from build123d import *

# Parameters (mm, degrees)
F0_W          = 100
F0_H          = 30
F1_DEPTH      = 30
F3_R          = 10.5
F4_DEPTH      = 100
F5_W          = 30
F5_H          = 30
F6_DEPTH      = 35
F2_W          = 30
F2_H          = 30
F7_DEPTH      = 35
F9_DEPTH      = 5
F10_DEPTH     = 35
F11_DEPTH     = 30
F12_DEPTH     = 5
F13_R         = 10.5
F14_DEPTH     = 50
F15_R         = 10.5
F16_DEPTH     = 50
F17_T4_DEPTH  = 78.1749423251
F17_T9_DEPTH  = 78.1749423251
F17_T14_DEPTH = 60.7168298797
F17_T19_DEPTH = 60.7168298797
F18_T4_DEPTH  = 52.8584149398
F18_T9_DEPTH  = 60.7168298797
F18_T15_DEPTH = 60.7168298797
F18_T21_DEPTH = 60.7168298797
F18_T27_DEPTH = 60.7168298797
F18_T33_DEPTH = 52.8584149398


# Not quite as in the source:
# - a fillet or chamfer that OpenCascade refuses, or shapes differently, is made with other operations: its cross-section is extruded or revolved along the edge and cut away or added


with BuildPart() as f1:
    # F0 (on Top) → F1 (new body)
    with BuildSketch(Plane.XY):
        Rectangle(F0_W, F0_H)
    extrude(amount=F1_DEPTH)

    # F3 (on face) → F4 (cut)
    with BuildSketch(Plane(origin=(-50, 0, 0), x_dir=(0, -1, 0), z_dir=(-1, 0, 0))):
        with Locations((0, 15)):
            Circle(F3_R)
    extrude(amount=-F4_DEPTH, mode=Mode.SUBTRACT)

    # F5 (on face) → F6 (join)
    with BuildSketch(Plane.XZ.offset(15)):
        with Locations((0, 15)):
            Rectangle(F5_W, F5_H)
    extrude(amount=F6_DEPTH)

    # F2 (on face) → F7 (join)
    with BuildSketch(Plane.XY.offset(30)):
        Rectangle(F2_W, F2_H)
    extrude(amount=F7_DEPTH)

    # F8 (on face) → F9 (join)
    with BuildSketch(Plane(origin=(-15, 0, 0), x_dir=(0, -1, 0), z_dir=(-1, 0, 0))):
        Polygon((15, 65), (15, 30), (24.8667589854, 63.5804566247), (-2.7490875563, 71.6946673709), (-4.7161444721, 65), align=None)
        Polygon((-15, 30), (15, 30), (15, 65), (-4.7161444721, 65), align=None)
    extrude(amount=F9_DEPTH)

    # F10 (cut, through all): a face of the model
    f10_faces = [f1.faces().sort_by_distance(p)[0] for p in [
        (0, 0, 65),
    ]]
    extrude(f10_faces, amount=-F10_DEPTH, mode=Mode.SUBTRACT)

    # F8 (on face) → F11 (join)
    with BuildSketch(Plane(origin=(-15, 0, 0), x_dir=(0, -1, 0), z_dir=(-1, 0, 0))):
        Polygon((-15, 30), (15, 30), (15, 65), (-4.7161444721, 65), align=None)
        Polygon((15, 65), (15, 30), (24.8667589854, 63.5804566247), (-2.7490875563, 71.6946673709), (-4.7161444721, 65), align=None)
    extrude(amount=-F11_DEPTH)

    # F12 (cut): a face of the model
    f12_faces = [f1.faces().sort_by_distance(p)[0] for p in [
        (-20, -5.0118640534, 48.8916696379),
    ]]
    extrude(f12_faces, amount=-F12_DEPTH, mode=Mode.SUBTRACT)

    # F13 (on face) → F14 (cut)
    with BuildSketch(Plane.XZ.offset(50)):
        with Locations((0, 15)):
            Circle(F13_R)
    extrude(amount=-F14_DEPTH, mode=Mode.SUBTRACT)

    # F15 (on face) → F16 (cut)
    with BuildSketch(Plane(origin=(0, -19.1730464608, 65.2534085396), x_dir=(1, 0, 0), z_dir=(0, -0.2819073996, 0.9594416178))):
        with Locations((0, 8.4572219875)):
            Circle(F15_R)
    extrude(amount=-F16_DEPTH, mode=Mode.SUBTRACT)

    # F17: chamfer of 5 on 4 edges, made by hand


with BuildPart() as f17_tool2:
    # F17_s3 → F17_t4 (new body)
    with BuildSketch(Plane(origin=(0, -22.7979287792, 77.5903069724), x_dir=(1, 0, 0), z_dir=(0, 0.2819073996, -0.9594416178))):
        Polygon((-10, -22.8488462553), (-15, -17.8488462553), (-15, -22.8488462553), align=None)
    extrude(amount=F17_T4_DEPTH)

    split(bisect_by=Plane.XY.offset(30), keep=Keep.TOP)


with BuildPart() as f1_1:
    add(f1.part)

    # F17_t1: cut F17_tool2
    add(f17_tool2.part, mode=Mode.SUBTRACT)


with BuildPart() as f17_tool7:
    # F17_s8 → F17_t9 (new body)
    with BuildSketch(Plane(origin=(0, -22.7979287792, 77.5903069724), x_dir=(1, 0, 0), z_dir=(0, 0.2819073996, -0.9594416178))):
        Polygon((15, -17.8488462553), (10, -22.8488462553), (15, -22.8488462553), align=None)
    extrude(amount=F17_T9_DEPTH)

    split(bisect_by=Plane.XY.offset(30), keep=Keep.TOP)


with BuildPart() as f1_2:
    add(f1_1.part)

    # F17_t6: cut F17_tool7
    add(f17_tool7.part, mode=Mode.SUBTRACT)


with BuildPart() as f17_tool12:
    # F17_s13 → F17_t14 (new body)
    with BuildSketch(Plane(origin=(0, -5.6814051569, 19.3360534821), x_dir=(1, 0, 0), z_dir=(0, -0.2819073996, 0.9594416178))):
        Polygon((15, -0.9344022802), (10, -5.9344022802), (15, -5.9344022802), align=None)
    extrude(amount=F17_T14_DEPTH)

    split(bisect_by=Plane.XY.offset(30), keep=Keep.TOP)


with BuildPart() as f1_3:
    add(f1_2.part)

    # F17_t11: cut F17_tool12
    add(f17_tool12.part, mode=Mode.SUBTRACT)


with BuildPart() as f17_tool17:
    # F17_s18 → F17_t19 (new body)
    with BuildSketch(Plane(origin=(0, -5.6814051569, 19.3360534821), x_dir=(1, 0, 0), z_dir=(0, -0.2819073996, 0.9594416178))):
        Polygon((-10, -5.9344022802), (-15, -0.9344022802), (-15, -5.9344022802), align=None)
    extrude(amount=F17_T19_DEPTH)

    split(bisect_by=Plane.XY.offset(30), keep=Keep.TOP)


with BuildPart() as f1_4:
    add(f1_3.part)

    # F17_t16: cut F17_tool17
    add(f17_tool17.part, mode=Mode.SUBTRACT)

    # F18: chamfer of 5 on 6 edges, made by hand


with BuildPart() as f18_tool2:
    # F18_s3 → F18_t4 (new body)
    with BuildSketch(Plane.YZ.offset(62.8584149398)):
        Polygon((10, 30), (15, 25), (15, 30), align=None)
    extrude(amount=-F18_T4_DEPTH)

    split(bisect_by=Plane(origin=(16.4244231276, 15.7582750978, 4.6301664136), x_dir=(-0.6923221184, 0.7215885839, 0), z_dir=(0.7071067812, 0.6784276741, 0.1993386339)), keep=Keep.TOP)


with BuildPart() as f1_5:
    add(f1_4.part)

    # F18_t1: cut F18_tool2
    add(f18_tool2.part, mode=Mode.SUBTRACT)


with BuildPart() as f18_tool7:
    # F18_s8 → F18_t9 (new body)
    with BuildSketch(Plane.YZ.offset(-2.1415850602)):
        Polygon((-10, 30), (-15, 25), (-15, 30), align=None)
    extrude(amount=-F18_T9_DEPTH)

    split(bisect_by=Plane(origin=(-7.9672011401, -7.6440643516, -2.2460129554), x_dir=(0.6923221184, -0.7215885839, 0), z_dir=(-0.7071067812, -0.6784276741, -0.1993386339)), keep=Keep.TOP)

    split(bisect_by=Plane(origin=(-20, 0, 20), x_dir=(0, 1, 0), z_dir=(-0.7071067812, 0, 0.7071067812)), keep=Keep.TOP)


with BuildPart() as f1_6:
    add(f1_5.part)

    # F18_t6: cut F18_tool7
    add(f18_tool7.part, mode=Mode.SUBTRACT)


with BuildPart() as f18_tool13:
    # F18_s14 → F18_t15 (new body)
    with BuildSketch(Plane.YZ.offset(2.1415850602)):
        Polygon((-15, 25), (-10, 30), (-15, 30), align=None)
    extrude(amount=F18_T15_DEPTH)

    split(bisect_by=Plane(origin=(7.9672011401, -7.6440643516, -2.2460129554), x_dir=(0.6923221184, 0.7215885839, 0), z_dir=(0.7071067812, -0.6784276741, -0.1993386339)), keep=Keep.TOP)

    split(bisect_by=Plane(origin=(20, 0, 20), x_dir=(0, 1, 0), z_dir=(0.7071067812, 0, 0.7071067812)), keep=Keep.TOP)


with BuildPart() as f1_7:
    add(f1_6.part)

    # F18_t12: cut F18_tool13
    add(f18_tool13.part, mode=Mode.SUBTRACT)


with BuildPart() as f18_tool19:
    # F18_s20 → F18_t21 (new body)
    with BuildSketch(Plane.XZ.offset(2.1415850602)):
        Polygon((-10, 30), (-15, 25), (-15, 30), align=None)
    extrude(amount=F18_T21_DEPTH)

    split(bisect_by=Plane(origin=(-7.9672011401, -7.6440643516, -2.2460129554), x_dir=(0.6923221184, -0.7215885839, 0), z_dir=(-0.7071067812, -0.6784276741, -0.1993386339)), keep=Keep.TOP)

    split(bisect_by=Plane(origin=(0, -20, 20), x_dir=(1, 0, 0), z_dir=(0, -0.7071067812, 0.7071067812)), keep=Keep.TOP)


with BuildPart() as f1_8:
    add(f1_7.part)

    # F18_t18: cut F18_tool19
    add(f18_tool19.part, mode=Mode.SUBTRACT)


with BuildPart() as f18_tool25:
    # F18_s26 → F18_t27 (new body)
    with BuildSketch(Plane.XZ.offset(2.1415850602)):
        Polygon((10, 30), (15, 25), (15, 30), align=None)
    extrude(amount=F18_T27_DEPTH)

    split(bisect_by=Plane(origin=(7.9672011401, -7.6440643516, -2.2460129554), x_dir=(0.6923221184, 0.7215885839, 0), z_dir=(0.7071067812, -0.6784276741, -0.1993386339)), keep=Keep.TOP)

    split(bisect_by=Plane(origin=(0, -20, 20), x_dir=(1, 0, 0), z_dir=(0, -0.7071067812, 0.7071067812)), keep=Keep.TOP)


with BuildPart() as f1_9:
    add(f1_8.part)

    # F18_t24: cut F18_tool25
    add(f18_tool25.part, mode=Mode.SUBTRACT)


with BuildPart() as f18_tool31:
    # F18_s32 → F18_t33 (new body)
    with BuildSketch(Plane.YZ.offset(-62.8584149398)):
        Polygon((10, 30), (15, 25), (15, 30), align=None)
    extrude(amount=F18_T33_DEPTH)

    split(bisect_by=Plane(origin=(-16.4244231276, 15.7582750978, 4.6301664136), x_dir=(-0.6923221184, -0.7215885839, 0), z_dir=(-0.7071067812, 0.6784276741, 0.1993386339)), keep=Keep.TOP)


with BuildPart() as f1_10:
    add(f1_9.part)

    # F18_t30: cut F18_tool31
    add(f18_tool31.part, mode=Mode.SUBTRACT)


solid = f1_10.part
Here's how the part is built. I have some questions about the finished solid (model axes, mm). A direction names the side the tool comes from. Coordinates: 2 decimals unless noted, no trailing zeros. Order: outer loops, then holes, each group sorted by start corner. A loop starts at its lowest first (then second) coordinate and runs counter-clockwise, first axis right, second up.
Item 1: If we section it at B-B on y = -31: List the corners of the cut face in (x, z) for me, plus the area to 3 significant figures.
Result sheet:
outline: (-15, 0) - (15, 0) - (15, 25) - (10, 30) - (-10, 30) - (-15, 25) - close; hole circle Ø21 at (0, 15)
area: 529 mm2
Item 2: For faces 4 (the face through (0, -32, 30)), 5 (the face through (15, -32, 12)), 6 (the face through (-12, -31, 28)), 7 (the face through (31, 12, 28)), 8 (the face through (15, -5, 50)), which set-ups out of +Z, -Z, +X, -X, +Y, -Y let a thin tool reach every point of the face, with its end or its side?
Result sheet:
face 4: +X, -X, -Y
face 5: +Z, -Z, +X, -Y
face 6: -X, -Y
face 7: +Z, +X, +Y
face 8: +Z, +X, +Y, -Y
Item 3: If we section it at C-C on y = -23.5: List the corners of the cut face in (x, z) for me.
Result sheet:
outline: (-15, 0) - (15, 0) - (15, 25) - (10, 30) - (-10, 30) - (-15, 25) - close; (-11.42, 63.98) - (-10, 58.93) - (10, 58.93) - (11.42, 63.98) - close; hole circle Ø21 at (0, 15)
Item 4: If we section it at A-A on z = 15: List the corners of the cut face in (x, y) for me, plus the area to 3 significant figures.
Result sheet:
outline: (-50, -15) - (-15, -15) - (-15, -50) - (-10.5, -50) - (-10.5, -10.5) - (-50, -10.5) - close; (-50, 10.5) - (50, 10.5) - (50, 15) - (-50, 15) - close; (10.5, -50) - (15, -50) - (15, -15) - (50, -15) - (50, -10.5) - (10.5, -10.5) - close
area: 1,120 mm2
Item 5: For P1, Ø6, axis at x = 26, y = 5, coming from the +Z side; P2, Ø4, axis at y = -2.5, z = 37.5, coming from the +X side; P3, Ø10, axis at x = 29, z = 14.5, coming from the -Y side, each with a flat end and sliding along its axis, tell me the tip position at first contact or that it passes through.
Result sheet:
P1: stops at z = 30
P2: stops at x = 15
P3: stops at y = -15
Item 6: I need wall thicknesses on line 1 (Z direction, x = 0, y = -39); line 2 (X direction, y = -33, z = 15); line 3 (Y direction, x = 20, z = 6.5). Which ranges of each line are inside material? Lowest first, please.
Result sheet:
line 1: z = 0 to 4.5, 25.5 to 30
line 2: x = -15 to -10.5, 10.5 to 15
line 3: y = -15 to -6.16, 6.16 to 15
Item 7: If we mould it in two halves opening along Z, with no side actions, what happens to faces 1 (the face through (-0.1, 10.3, 21.8)), 2 (the face through (-1, -10, 0)), 3 (the face through (-33, -15, 12))? For each: +Z half, -Z half, draft (parallel to the pull), parting line (faces both ways), or undercut.
Result sheet:
face 1: undercut
face 2: -Z half
face 3: draft
